Geometry: final body of the model. Coordinates: model frame, mm. Face numbers are marked on the shaded views. A direction names the side the tool comes from. Coordinates: 2 decimals unless noted, no trailing zeros. Loops run counter-clockwise (first coordinate to the right, second up) from the corner with the lowest first, then second, coordinate; pieces in that order, holes last. Notation, with made-up numbers: M -15.5,-14.75 L 1.5,-14.75 A38 cw 1.5,24.25 Z; hole C 24,28 d8. An arc over 180 degrees is marked long. Write item = value, one per line. Start each with the question number.
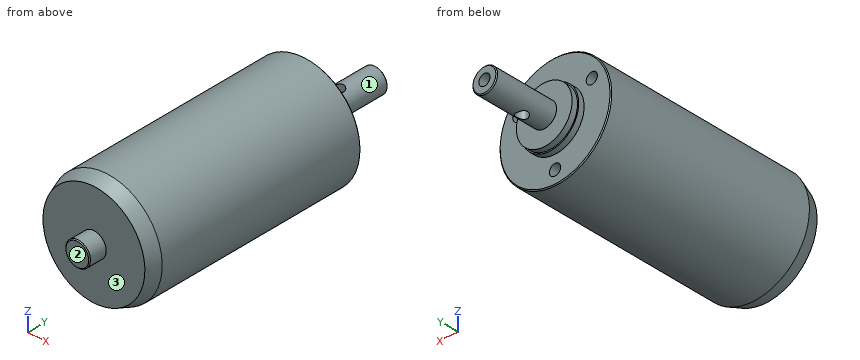
```python
from build123d import *

# Parameters (mm, degrees)
CHAMFER_1_SIZE         = 0.2
CHAMFER_2_SIZE         = 3
CHAMFER_2_SIZE2        = 1.091910703
HOLE_WIZARD_M3_1_D     = 2.5
HOLE_WIZARD_M3_1_DEPTH = 5.5
HOLE_WIZARD_M3_1_TIP   = 0.751075774
HOLE_WIZARD_M3_2_D     = 2.5
HOLE_WIZARD_M3_2_DEPTH = 7.5
HOLE_WIZARD_M3_2_TIP   = 0.751075774
HOLE_WIZARD_M3_3_D     = 2.5
HOLE_WIZARD_M3_3_DEPTH = 4
HOLE_WIZARD_M3_3_TIP   = 0.751075774


with BuildPart() as part:
    # 草图1 → 旋转1 (revolve)
    with BuildSketch(Plane(origin=(0, 0, 0), x_dir=(0, 0, -1), z_dir=(1, 0, 0)), mode=Mode.PRIVATE) as revolve_1_sk:
        Polygon((0, 0), (2.75, 0), (2.75, 4), (12.5, 4), (12.5, 54.8), (6.5, 54.8), (6.5, 56.1), (6.238591707, 56.1), (6.238591707, 57.4), (2.75, 57.4), (2.75, 71.8), (0, 71.8), align=None)
    revolve(revolve_1_sk.sketch.rotate(Axis((0, 90.041930378, 0), (0, -1, 0)), 180), axis=Axis((0, 90.041930378, 0), (0, -1, 0)))

    # 倒角1
    chamfer_1_edges = [part.edges().sort_by_distance(p)[0] for p in [
        (0, 54.8, -12.5),
        (0, 0, -2.75),
        (0, 71.8, -2.75),
    ]]
    chamfer(chamfer_1_edges, length=CHAMFER_1_SIZE)

    # 倒角2
    chamfer_2_edges = [part.edges().sort_by_distance(p)[0] for p in [
        (0, 4, -12.5),
    ]]
    chamfer_2_side = [part.faces().sort_by_distance(p)[0] for p in [
        (0, 29.3, -12.5),
    ]]
    chamfer(chamfer_2_edges, length=CHAMFER_2_SIZE, length2=CHAMFER_2_SIZE2, reference=chamfer_2_side[0])

    # M3 螺纹孔1
    with Locations(Plane(origin=(0, 71.8, 0), x_dir=(1, 0, 0), z_dir=(0, 1, 0))):
        with Locations((0, 0)):
            Hole(HOLE_WIZARD_M3_1_D / 2, depth=HOLE_WIZARD_M3_1_DEPTH)
            with Locations((0, 0, -(HOLE_WIZARD_M3_1_DEPTH + HOLE_WIZARD_M3_1_TIP / 2))):  # 118° drill point
                Cone(0, HOLE_WIZARD_M3_1_D / 2, HOLE_WIZARD_M3_1_TIP, mode=Mode.SUBTRACT)

    # M3 螺纹孔2
    with Locations(Plane.XY.offset(2.75)):
        with Locations((0, 62.8)):
            Hole(HOLE_WIZARD_M3_2_D / 2, depth=HOLE_WIZARD_M3_2_DEPTH)
            with Locations((0, 0, -(HOLE_WIZARD_M3_2_DEPTH + HOLE_WIZARD_M3_2_TIP / 2))):  # 118° drill point
                Cone(0, HOLE_WIZARD_M3_2_D / 2, HOLE_WIZARD_M3_2_TIP, mode=Mode.SUBTRACT)

    # M3 螺纹孔3
    with Locations(Plane(origin=(0, 54.8, 0), x_dir=(1, 0, 0), z_dir=(0, 1, 0))):
        with Locations((0, 9.5), (-8.227241336, -4.75), (8.227241336, -4.75)):
            Hole(HOLE_WIZARD_M3_3_D / 2, depth=HOLE_WIZARD_M3_3_DEPTH)
            with Locations((0, 0, -(HOLE_WIZARD_M3_3_DEPTH + HOLE_WIZARD_M3_3_TIP / 2))):  # 118° drill point
                Cone(0, HOLE_WIZARD_M3_3_D / 2, HOLE_WIZARD_M3_3_TIP, mode=Mode.SUBTRACT)


solid = part.part
```
Item 1: Section query A-A (y = 59). Return the cut outline in (x, z), plus the area to 3 significant figures.
Item 2: Section query B-B (y = 31). Return the cut outline in (x, z).
Item 3: Line query: line 1 (X direction, y = 62.8, z = 0.25); line 2 (Y direction, x = 0, z = -1.45); line 3 (Y direction, x = 4.25, z = 0.25). Output: solid intervals per line, ascending. Write a range as from..to.
Item 4: First-contact query: pin 1 (4 mm diameter, centred on y = 51, z = -9, fed in from +X); pin 2 (12 mm diameter, centred on y = 30.5, z = -9.5, fed in from +X); pin 3 (3 mm diameter, centred on x = 2, z = -8.5, fed in from +Y). Flat tips, straight axial feed; report the tip coordinate or a pass-through.
Item 5: Reachability of the marked faces 1, 2 and 3 from +Z, -Z, +X, -X, +Y, -Y: full face, straight path, thin tool, end or side. Return the list, or none.
Verdict:
q1.outline = C 0,0 d5.5
q1.area = 23.8 mm2
q2.outline = C 0,0 d25
q3.line_1 = -2.74..-1.25, 1.25..2.74
q3.line_2 = 0..61.55, 64.05..71.8
q3.line_3 = 4..57.4
q4.pin_1 = 10.36
q4.pin_2 = 12
q4.pin_3 = 54.8
q5.face_1 = +Y
q5.face_2 = +Z, -Z, +X, -X, -Y
q5.face_3 = -Y
